Could you check a few things on this model? Use its own coordinates, in mm. Face numbers are marked on the shaded views. A direction names the side the tool comes from. Give positions to 0.01 mm unless a question says otherwise; leave off trailing zeros. Loops run counter-clockwise (first coordinate to the right, second up) from the corner with the lowest first, then second, coordinate; pieces in that order, holes last. Notation, with made-up numbers: (-40, 80) - (-8, 80) arc R10 ccw to (-8, 93) - close; hole circle Ø6 at (-30.75, 29). An arc over 180 degrees is marked (long way). Use CSV: the item, a comma, the result in double quotes.
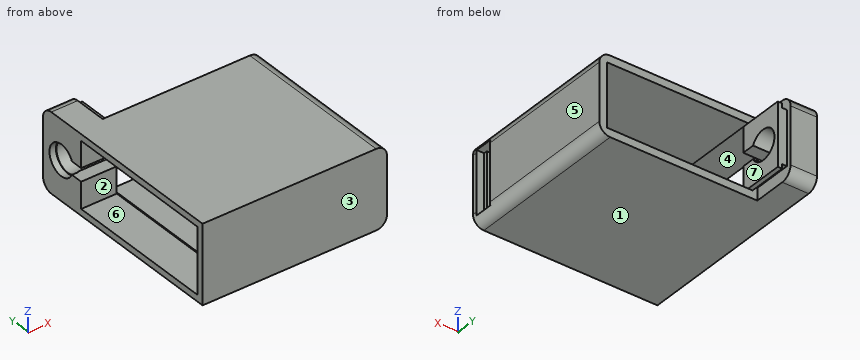
from build123d import *

# Parameters (mm, degrees)
SKETCH_1_W           = 72.2
SKETCH_1_H           = 36.2
SKETCH_1_W_2         = 65
SKETCH_1_H_2         = 29
EXTRUDE_1_DEPTH      = 74.2
SKETCH_2_W           = 72.2
SKETCH_2_H           = 36.2
EXTRUDE_2_DEPTH      = 2
SKETCH_3_W           = 36.2
SKETCH_3_H           = 76.2
SKETCH_3_W_2         = 30.2
SKETCH_3_H_2         = 70.2
EXTRUDE_2_2_DEPTH    = 16.4
SKETCH_4_W           = 30.2
SKETCH_4_H           = 70.2
CUT_EXTRUDE_1_DEPTH  = 16.4
SKETCH_5_W           = 29
SKETCH_5_H           = 4.8
CUT_EXTRUDE_2_DEPTH  = 5
SKETCH_8_W           = 36.2
SKETCH_8_H           = 20
EXTRUDE_3_DEPTH      = 16.4
SKETCH_7_W           = 6
SKETCH_7_H           = 17
CUT_EXTRUDE_3_DEPTH  = 17
SKETCH_9_W           = 6
SKETCH_9_H           = 17
EXTRUDE_4_DEPTH      = 2
SKETCH_10_R          = 7.1
CUT_EXTRUDE_4_DEPTH  = 3
SKETCH_11_W          = 2.2
SKETCH_11_H          = 20
CUT_EXTRUDE_5_DEPTH  = 5.6
SKETCH_12_W          = 2.2
SKETCH_12_H          = 20
CUT_EXTRUDE_6_DEPTH  = 5.6
SKETCH_13_W          = 2
SKETCH_13_H          = 3.6
CUT_EXTRUDE_7_DEPTH  = 20
FILLET_1_R           = 5
FILLET_2_R           = 5
FILLET_3_R           = 5
FILLET_4_R           = 5
SKETCH_14_W          = 4.2
SKETCH_14_H          = 29
CUT_EXTRUDE_8_DEPTH  = 2.2
SKETCH_15_R          = 6.8
CUT_EXTRUDE_9_DEPTH  = 20
SKETCH_16_W          = 6
SKETCH_16_H          = 5.564939783
CUT_EXTRUDE_10_DEPTH = 10
SKETCH_17_W          = 65
SKETCH_17_H          = 29
EXTRUDE_5_DEPTH      = 1.6
SKETCH_18_W          = 3.6
SKETCH_18_H          = 29
CUT_EXTRUDE_11_DEPTH = 3.4
SKETCH_20_W          = 22.2
SKETCH_20_H          = 5
EXTRUDE_6_DEPTH      = 5.4


with BuildPart() as part:
    # 草图1 → 拉伸-薄壁1 (new body)
    with BuildSketch(Plane(origin=(0, 0, 0), x_dir=(1, 0, 0), z_dir=(0, 1, 0))):
        with Locations((32.5, 14.5)):
            Rectangle(SKETCH_1_W, SKETCH_1_H)
        with Locations((32.5, 14.5)):
            Rectangle(SKETCH_1_W_2, SKETCH_1_H_2, mode=Mode.SUBTRACT)
    extrude(amount=EXTRUDE_1_DEPTH)

    # 草图2 → Extrude 2 (add)
    with BuildSketch(Plane(origin=(0, 0, 0), x_dir=(1, 0, 0), z_dir=(0, 1, 0))):
        with Locations((32.5, 14.5)):
            Rectangle(SKETCH_2_W, SKETCH_2_H)
    extrude(amount=-EXTRUDE_2_DEPTH)

    # 草图3 → Extrude 2 2 (add)
    with BuildSketch(Plane(origin=(0, 0, 0), x_dir=(0, 0, -1), z_dir=(1, 0, 0))):
        with Locations((14.5, 36.1)):
            Rectangle(SKETCH_3_W, SKETCH_3_H)
        with Locations((14.5, 36.1)):
            Rectangle(SKETCH_3_W_2, SKETCH_3_H_2, mode=Mode.SUBTRACT)
    extrude(amount=-EXTRUDE_2_2_DEPTH)

    # 草图4 → 切除-拉伸1 (cut)
    with BuildSketch(Plane(origin=(0, 0, 0), x_dir=(0, 0, -1), z_dir=(1, 0, 0))):
        with Locations((14.5, 36.1)):
            Rectangle(SKETCH_4_W, SKETCH_4_H)
    extrude(amount=-CUT_EXTRUDE_1_DEPTH, mode=Mode.SUBTRACT)

    # 草图5 → 切除-拉伸2 (cut)
    with BuildSketch(Plane(origin=(68.6, 0, 0), x_dir=(0, 0, -1), z_dir=(1, 0, 0))):
        with Locations((14.5, 2.4)):
            Rectangle(SKETCH_5_W, SKETCH_5_H)
    extrude(amount=-CUT_EXTRUDE_2_DEPTH, mode=Mode.SUBTRACT)

    # 草图8 → 凸台-拉伸3 (add)
    with BuildSketch(Plane.ZY.offset(16.4)):
        with Locations((-14.5, 84.2)):
            Rectangle(SKETCH_8_W, SKETCH_8_H)
    extrude(amount=-EXTRUDE_3_DEPTH)

    # 草图7 → 切除-拉伸3 (cut)
    with BuildSketch(Plane(origin=(0, 0, 0), x_dir=(0, 0, -1), z_dir=(1, 0, 0))):
        with Locations((14.5, 79.7)):
            Rectangle(SKETCH_7_W, SKETCH_7_H)
    extrude(amount=-CUT_EXTRUDE_3_DEPTH, mode=Mode.SUBTRACT)

    # 草图9 → 凸台-拉伸4 (add)
    with BuildSketch(Plane.ZY.offset(16.4)):
        with Locations((-14.5, 79.7)):
            Rectangle(SKETCH_9_W, SKETCH_9_H)
    extrude(amount=-EXTRUDE_4_DEPTH)

    # 草图10 → 切除-拉伸4 (cut)
    with BuildSketch(Plane.ZY.offset(16.4)):
        with Locations((-14.5, 83.2)):
            Circle(SKETCH_10_R)
    extrude(amount=-CUT_EXTRUDE_4_DEPTH, mode=Mode.SUBTRACT)

    # 草图11 → 切除-拉伸5 (cut)
    with BuildSketch(Plane.XY.offset(3.6)):
        with Locations((-3.1, 84.2)):
            Rectangle(SKETCH_11_W, SKETCH_11_H)
    extrude(amount=-CUT_EXTRUDE_5_DEPTH, mode=Mode.SUBTRACT)

    # 草图12 → 切除-拉伸6 (cut)
    with BuildSketch(Plane(origin=(0, 0, -32.6), x_dir=(-1, 0, 0), z_dir=(0, 0, -1))):
        with Locations((3.1, 84.2)):
            Rectangle(SKETCH_12_W, SKETCH_12_H)
    extrude(amount=-CUT_EXTRUDE_6_DEPTH, mode=Mode.SUBTRACT)

    # 草图13 → 切除-拉伸7 (cut)
    with BuildSketch(Plane(origin=(0, 94.2, 0), x_dir=(1, 0, 0), z_dir=(0, 1, 0))):
        with Locations((-1, 30.8)):
            Rectangle(SKETCH_13_W, SKETCH_13_H)
        with Locations((-1, -1.8)):
            Rectangle(SKETCH_13_W, SKETCH_13_H)
    extrude(amount=-CUT_EXTRUDE_7_DEPTH, mode=Mode.SUBTRACT)

    # 圆角1
    fillet_1_edges = [part.edges().sort_by_distance(p)[0] for p in [
        (-10.3, 94.2, 3.6),
    ]]
    fillet(fillet_1_edges, radius=FILLET_1_R)

    # 圆角2
    fillet_2_edges = [part.edges().sort_by_distance(p)[0] for p in [
        (-10.3, 94.2, -32.6),
    ]]
    fillet(fillet_2_edges, radius=FILLET_2_R)

    # 圆角3
    # the kernel refuses this fillet: 5 mm, written as the material it takes off along each edge
    with BuildSketch(Plane(origin=(68.6, -14.5, 3.6), x_dir=(-1, 0, 0), z_dir=(0, 1, 0))) as fillet_3_piece_1:
        with BuildLine():
            CenterArc((FILLET_3_R, -FILLET_3_R), FILLET_3_R, 90, 90)
            Line((0, -FILLET_3_R), (0, 0))
            Line((0, 0), (FILLET_3_R, 0))
        make_face()
    extrude(amount=101.2, mode=Mode.SUBTRACT)

    # 圆角4
    # the kernel refuses this fillet: 5 mm, written as the material it takes off along each edge
    with BuildSketch(Plane(origin=(68.6, -14.5, -32.6), x_dir=(-1, 0, 0), z_dir=(0, 1, 0))) as fillet_4_piece_1:
        with BuildLine():
            CenterArc((FILLET_4_R, FILLET_4_R), FILLET_4_R, 180, 90)
            Line((0, FILLET_4_R), (0, 0))
            Line((0, 0), (FILLET_4_R, 0))
        make_face()
    extrude(amount=101.2, mode=Mode.SUBTRACT)

    # 草图14 → 切除-拉伸8 (cut)
    with BuildSketch(Plane(origin=(0, 94.2, 0), x_dir=(1, 0, 0), z_dir=(0, 1, 0))):
        with Locations((-2.1, 14.5)):
            Rectangle(SKETCH_14_W, SKETCH_14_H)
    extrude(amount=-CUT_EXTRUDE_8_DEPTH, mode=Mode.SUBTRACT)

    # 草图15 → 切除-拉伸9 (cut)
    with BuildSketch(Plane.ZY.offset(13.4)):
        with Locations((-14.5, 83.2)):
            Circle(SKETCH_15_R)
    extrude(amount=-CUT_EXTRUDE_9_DEPTH, mode=Mode.SUBTRACT)

    # 草图16 → 切除-拉伸10 (cut)
    with BuildSketch(Plane(origin=(-14.4, 0, 0), x_dir=(0, 0, -1), z_dir=(1, 0, 0))):
        with Locations((14.5, 73.982469892)):
            Rectangle(SKETCH_16_W, SKETCH_16_H)
    extrude(amount=-CUT_EXTRUDE_10_DEPTH, mode=Mode.SUBTRACT)

    # 草图17 → 凸台-拉伸5 (add)
    with BuildSketch(Plane(origin=(0, 0, 0), x_dir=(1, 0, 0), z_dir=(0, 1, 0))):
        with Locations((32.5, 14.5)):
            Rectangle(SKETCH_17_W, SKETCH_17_H)
    extrude(amount=EXTRUDE_5_DEPTH)

    # 草图18 → 切除-拉伸11 (cut)
    with BuildSketch(Plane.XZ.offset(-4.8)):
        with Locations((66.8, -14.5)):
            Rectangle(SKETCH_18_W, SKETCH_18_H)
    extrude(amount=-CUT_EXTRUDE_11_DEPTH, mode=Mode.SUBTRACT)

    # 草图20 → 凸台-拉伸6 (add)
    with BuildSketch(Plane(origin=(65, 0, 0), x_dir=(0, 0, -1), z_dir=(1, 0, 0))):
        with Locations((14.5, 9.1)):
            Rectangle(SKETCH_20_W, SKETCH_20_H)
    extrude(amount=-EXTRUDE_6_DEPTH)


solid = part.part
1) Suppose I cut it at B-B (z = -5.5). Please give me the cut outline in (x, y).
Answer below:
outline,"(-16.4, -2) - (68.6, -2) - (68.6, 0) - (65, 0) - (65, 1.6) - (0, 1.6) - (0, 1) - (-16.4, 1) - close; (-16.4, 71.2) - (0, 71.2) - (0, 92) - (-4.2, 92) - (-4.2, 94.2) - (-16.4, 94.2) - close; (59.6, 6.6) - (65, 6.6) - (65, 8.2) - (68.6, 8.2) - (68.6, 74.2) - (65, 74.2) - (65, 11.6) - (59.6, 11.6) - close"
2) Suppose I cut it at A-A (y = 83.2). Please give me the cut outline in (x, z), plus the area to 3 significant figures.
Answer below:
outline,"(-16.4, -32.6) - (-4.2, -32.6) - (-4.2, -27) - (-2, -27) - (-2, -29) - (0, -29) - (0, -21.3) - (-13.4, -21.3) - (-13.4, -21.6) - (-16.4, -21.6) - close; (-16.4, -7.4) - (-13.4, -7.4) - (-13.4, -7.7) - (0, -7.7) - (0, 0) - (-2, 0) - (-2, -2) - (-4.2, -2) - (-4.2, 3.6) - (-16.4, 3.6) - close"
area,"330 mm2"
3) Suppose I cut it at D-D (z = -14.5). Please give me the cut outline in (x, y).
Answer below:
outline,"(-16.4, -2) - (68.6, -2) - (68.6, 0) - (65, 0) - (65, 1.6) - (0, 1.6) - (0, 1) - (-16.4, 1) - close; (-16.4, 90.3) - (-13.4, 90.3) - (-13.4, 90) - (0, 90) - (0, 92) - (-4.2, 92) - (-4.2, 94.2) - (-16.4, 94.2) - close; (59.6, 6.6) - (65, 6.6) - (65, 8.2) - (68.6, 8.2) - (68.6, 74.2) - (65, 74.2) - (65, 11.6) - (59.6, 11.6) - close"
4) I'm going to push flat-ended pins straight in: P1, Ø3.5, axis at x = -3, z = -13.5, coming from the +Y side; P2, Ø1.1, axis at x = -3.5, y = 80.5, coming from the +Z side; P3, Ø6, axis at y = 27.5, z = -13.5, coming from the -X side; P4, Ø5.5, axis at y = 8.5, z = -10, coming from the -X side. Where does each tip first touch, or does it pass through?
Answer below:
P1,"stops at y = 94.2"
P2,"stops at z = -2"
P3,"stops at x = 65"
P4,"stops at x = 59.6"
5) I need wall thicknesses on line 1 along Y through (x, z) = (-3.75, -14.5); line 2 along Y through (x, z) = (-2, -6); line 3 along Z through (x, y) = (-2, 29). Which ranges of each line are inside material? Lowest first, please.
Answer below:
line 1,"y = -2 to 1, 90 to 92"
line 2,"y = -2 to 1, 71.2 to 92"
line 3,"z = -32.6 to -29.6, 0.6 to 3.6"
6) Which directions (+Z, -Z, +X, -X, +Y, -Y) give clear straight access to the entire face, cutting with the end or side of a thin tool? Please do the marked faces 5, 6 and 7.
Answer below:
face 5,"+Z, -Z, +X, +Y, -Y"
face 6,"-X"
face 7,"+Y"
7) Suppose I cut it at C-C (y = 33). Please give me the cut outline in (x, z).
Answer below:
outline,"(-16.4, -32.6) - (63.6, -32.6) arc R5 ccw to (68.6, -27.6) - (68.6, -1.4) arc R5 ccw to (63.6, 3.6) - (-16.4, 3.6) - (-16.4, 0.6) - (0, 0.6) - (0, 0) - (65, 0) - (65, -29) - (0, -29) - (0, -29.6) - (-16.4, -29.6) - close"
8) We'd pull the mould along Y, two halves only. Please class the marked faces 1, 2, 3 and 4: +Y half, -Y half, draft (parallel to the pull), parting line (faces both ways), or undercut.
Answer below:
face 1,"draft"
face 2,"undercut"
face 3,"-Y half"
face 4,"undercut"
